For this review, take the finished solid that the model builds, in its own axes (mm). A direction names the side the tool comes from. Give positions to 0.01 mm unless a question says otherwise; leave off trailing zeros. Order: outer loops, then holes, each group sorted by start corner. A loop starts at its lowest first (then second) coordinate and runs counter-clockwise, first axis right, second up. Notation, with made-up numbers: (-39.75, -34.75) - (14.25, -34.75) arc R21 cw to (14.25, -28.75) - close; hole circle Ø8 at (0.25, -18.5). An arc over 180 degrees is marked (long way). Use a Markdown table: item, result. Add a question column.
1) Machinability: for faces 1 (the face through (34, -25.4, 25)), 2 (the face through (35, 10, -18.469)), 3 (the face through (-35.56, -2, 14)), 4 (the face through (36.068, -14, 6)), which of the approach directions +Z, -Z, +X, -X, +Y, -Y give a long, thin tool a straight path to every point of the face, cutting with its end or side? Answer none if there is none.
2) Wall thickness on L1, parallel to X at y = 0, z = 8.5; L2, parallel to X at y = 20, z = 22; L3, parallel to X at y = -22, z = -12: over which ranges is each line inside the solid? List them lowest first.
3) We need section B-B on x = 30. Write out the cut boundary in (y, z), then the cut area to 3 significant figures.
4) We need section A-A on z = 5.5. Write out the cut boundary in (x, y), then the cut area to 3 significant figures.
5) Clearance check with flat-ended pins moving along their axes: P1, Ø1.5, axis at x = 11, y = 3.5, coming from the -Z side; P2, Ø1, axis at y = 13.5, z = 21.5, coming from the +X side; P3, Ø9.5, axis at y = -17.5, z = 12.5, coming from the -X side. State where each tip first meets the part, or that it passes through.
6) Mouldability with a two-part tool opening along Y and no side actions: class faces 5 (the face through (-36, -27.94, 5)), 6 (the face through (-1, 17, 29.791)), 7 (the face through (35.56, -24, -20)) as released by +Y, released by -Y, zero draft, split by the parting line, or undercut.
```python
from build123d import *

# Parameters (mm, degrees)
F0_W          = 76.2
F0_H          = 50.8
F1_DEPTH      = 25.4
F1_DEPTH_BACK = 25.4
F2_W          = 71.12
F2_H          = 50.8
F3_DEPTH      = 25.4
F4_W          = 71.12
F4_H          = 48.26
F5_DEPTH      = 22.86
F6_W          = 48.26
F6_H          = 2.54
F7_DEPTH      = 2.54
F8_W          = 48.26
F8_H          = 2.54
F9_DEPTH      = 2.54
F10_W         = 48.26
F10_H         = 2.54
F11_DEPTH     = 2.54
F12_W         = 48.26
F12_H         = 2.54
F13_DEPTH     = 2.54
F15_W         = 1.27
F15_H         = 1.27
F16_DEPTH     = 48.26
F17_W         = 1.27
F17_H         = 1.27
F18_DEPTH     = 48.26
F19_W         = 1.27
F19_H         = 1.2642855102
F20_DEPTH     = 48.26
F21_W         = 1.27
F21_H         = 1.27
F22_DEPTH     = 48.26
F23_W         = 1.27
F23_H         = 1.27
F24_DEPTH     = 48.26
F25_W         = 1.27
F25_H         = 1.27
F26_DEPTH     = 48.26
F27_W         = 1.27
F27_H         = 1.27
F28_DEPTH     = 48.26
F29_W         = 1.27
F29_H         = 1.27
F30_DEPTH     = 48.26
F31_W         = 5.08
F31_H         = 50.8
F32_DEPTH     = 2.794
F33_W         = 5.08
F33_H         = 50.8
F34_DEPTH     = 2.54
F35_W         = 18.5524672455
F35_H         = 50.8
F35_W_2       = 19.8015327545
F36_DEPTH     = 2.032
F37_W         = 18.5524672455
F37_H         = 2.54
F38_DEPTH     = 74.169
F39_W         = 19.8015327545
F39_H         = 2.5402396598
F40_DEPTH     = 74.169


# Not quite as in the source:
# - a pattern or mirror of a feature is missing from the dataset's text; its kind, count and spacing are read off the source's solid


with BuildPart() as f1:
    # F0 (on Front) → F1 (new body, two sides)
    with BuildSketch(Plane.XZ) as f1_sk:
        with Locations((0, 4.3905831537)):
            Rectangle(F0_W, F0_H)
    extrude(amount=F1_DEPTH)
    extrude(f1_sk.sketch, amount=-F1_DEPTH_BACK)

    # F2 (on face) → F3 (cut)
    with BuildSketch(Plane.XZ.offset(25.4)):
        with Locations((0, 4.3905831537)):
            Rectangle(F2_W, F2_H)
    extrude(amount=-F3_DEPTH, mode=Mode.SUBTRACT)

    # F4 (on face) → F5 (cut)
    with BuildSketch(Plane.XZ):
        with Locations((0, 3.1205831537)):
            Rectangle(F4_W, F4_H)
    extrude(amount=-F5_DEPTH, mode=Mode.SUBTRACT)

    # F6 (on face) → F7 (join)
    with BuildSketch(Plane.YZ.offset(-35.56)):
        with Locations((-1.27, -17.1994168463)):
            Rectangle(F6_W, F6_H)
    extrude(amount=F7_DEPTH)

    # F8 (on face) → F9 (join)
    with BuildSketch(Plane.YZ.offset(-35.56)):
        with Locations((-1.27, -4.4994168463)):
            Rectangle(F8_W, F8_H)
    extrude(amount=F9_DEPTH)

    # F10 (on face) → F11 (join)
    with BuildSketch(Plane.YZ.offset(-35.56)):
        with Locations((-1.27, 8.2005831537)):
            Rectangle(F10_W, F10_H)
    extrude(amount=F11_DEPTH)

    # F12 (on face) → F13 (join)
    with BuildSketch(Plane.YZ.offset(-35.56)):
        with Locations((-1.27, 20.9005831537)):
            Rectangle(F12_W, F12_H)
    extrude(amount=F13_DEPTH)

    # F14: F1 across plane


with BuildPart() as f1_1:
    add(f1.part)
    add(f1.part.mirror(Plane.YZ))

    # F15 (on face) → F16 (cut)
    with BuildSketch(Plane.XZ.offset(25.4)):
        with Locations((-34.925, -16.5644168463)):
            Rectangle(F15_W, F15_H)
    extrude(amount=-F16_DEPTH, mode=Mode.SUBTRACT)

    # F17 (on face) → F18 (cut)
    with BuildSketch(Plane.XZ.offset(25.4)):
        with Locations((-34.925, -3.8644168463)):
            Rectangle(F17_W, F17_H)
    extrude(amount=-F18_DEPTH, mode=Mode.SUBTRACT)

    # F19 (on face) → F20 (cut)
    with BuildSketch(Plane.XZ.offset(25.4)):
        with Locations((-34.925, 8.8384403986)):
            Rectangle(F19_W, F19_H)
    extrude(amount=-F20_DEPTH, mode=Mode.SUBTRACT)

    # F21 (on face) → F22 (cut)
    with BuildSketch(Plane.XZ.offset(25.4)):
        with Locations((-34.925, 21.5355831537)):
            Rectangle(F21_W, F21_H)
    extrude(amount=-F22_DEPTH, mode=Mode.SUBTRACT)

    # F23 (on face) → F24 (cut)
    with BuildSketch(Plane.XZ.offset(25.4)):
        with Locations((34.925, 21.5355831537)):
            Rectangle(F23_W, F23_H)
    extrude(amount=-F24_DEPTH, mode=Mode.SUBTRACT)

    # F25 (on face) → F26 (cut)
    with BuildSketch(Plane.XZ.offset(25.4)):
        with Locations((34.925, 8.8355831537)):
            Rectangle(F25_W, F25_H)
    extrude(amount=-F26_DEPTH, mode=Mode.SUBTRACT)

    # F27 (on face) → F28 (cut)
    with BuildSketch(Plane.XZ.offset(25.4)):
        with Locations((34.925, -3.8644168463)):
            Rectangle(F27_W, F27_H)
    extrude(amount=-F28_DEPTH, mode=Mode.SUBTRACT)

    # F29 (on face) → F30 (cut)
    with BuildSketch(Plane.XZ.offset(25.4)):
        with Locations((34.925, -16.5644168463)):
            Rectangle(F29_W, F29_H)
    extrude(amount=-F30_DEPTH, mode=Mode.SUBTRACT)

    # F31 (on face) → F32 (join)
    with BuildSketch(Plane.XZ.offset(25.4)):
        with Locations((35.56, 4.3905831537)):
            Rectangle(F31_W, F31_H)
    extrude(amount=F32_DEPTH)

    # F33 (on face) → F34 (join)
    with BuildSketch(Plane.XZ.offset(25.4)):
        with Locations((-35.56, 4.3905831537)):
            Rectangle(F33_W, F33_H)
    extrude(amount=F34_DEPTH)

    # F35 (on face) → F36 (cut)
    with BuildSketch(Plane.YZ.offset(38.1)):
        with Locations((-13.8377663772, 4.3905831537)):
            Rectangle(F35_W, F35_H)
        with Locations((10.4192336228, 4.3905831537)):
            Rectangle(F35_W_2, F35_H)
    f36 = extrude(amount=-F36_DEPTH, mode=Mode.SUBTRACT)

    # F36_copies: F36 across plane
    add(f36.mirror(Plane(origin=(0, 0, 0), x_dir=(0, 0, -1), z_dir=(-1, 0, 0))), mode=Mode.SUBTRACT)

    # F37 (on face) → F38 (cut, through all)
    with BuildSketch(Plane.YZ.offset(36.068)):
        with Locations((-13.8377663772, -19.7394168463)):
            Rectangle(F37_W, F37_H)
    extrude(amount=-F38_DEPTH, mode=Mode.SUBTRACT)

    # F39 (on face) → F40 (cut, through all)
    with BuildSketch(Plane.YZ.offset(36.068)):
        with Locations((10.4192336228, -19.7392970164)):
            Rectangle(F39_W, F39_H)
    extrude(amount=-F40_DEPTH, mode=Mode.SUBTRACT)


solid = f1_1.part
```
Checked values:
| question | item | result |
|---|---|---|
| 1 | face 1 | +Z |
| 1 | face 2 | -Z, +X, -X |
| 1 | face 3 | none |
| 1 | face 4 | +Z, -Z, +X |
| 2 | L1 | -38.1 to -35.56, -34.29 to -33.02, 33.02 to 34.29, 35.56 to 38.1 |
| 2 | L2 | -36.07 to -35.56, -34.29 to -33.02, 33.02 to 34.29, 35.56 to 36.07 |
| 2 | L3 | -36.07 to -35.56, 35.56 to 36.07 |
| 3 | outline | (0, 27.25) - (22.86, 27.25) - (22.86, -21.01) - (25.4, -21.01) - (25.4, 29.79) - (0, 29.79) - close |
| 3 | area | 187 mm² |
| 4 | outline | (-38.1, -27.94) - (-33.02, -27.94) - (-33.02, -25.4) - (-35.56, -25.4) - (-35.56, 22.86) - (35.56, 22.86) - (35.56, -25.4) - (33.02, -25.4) - (33.02, -28.19) - (38.1, -28.19) - (38.1, -23.11) - (36.07, -23.11) - (36.07, -4.56) - (38.1, -4.56) - (38.1, 0.52) - (36.07, 0.52) - (36.07, 20.32) - (38.1, 20.32) - (38.1, 25.4) - (-38.1, 25.4) - (-38.1, 20.32) - (-36.07, 20.32) - (-36.07, 0.52) - (-38.1, 0.52) - (-38.1, -4.56) - (-36.07, -4.56) - (-36.07, -23.11) - (-38.1, -23.11) - close |
| 4 | area | 310 mm² |
| 5 | P1 | z = 27.25 |
| 5 | P2 | x = 36.07 |
| 5 | P3 | x = -36.07 |
| 6 | face 5 | released by -Y |
| 6 | face 6 | zero draft |
| 6 | face 7 | undercut |
